Design review of the part shown in the three views and the two pictorial views. Dimensions are in mm from the part's minimum x, y and z. Round coordinates to 2 decimals unless told otherwise and drop trailing zeros. Order: outer loops, then holes, each group sorted by start corner. A loop starts at its lowest first (then second) coordinate and runs counter-clockwise, first axis right, second up.
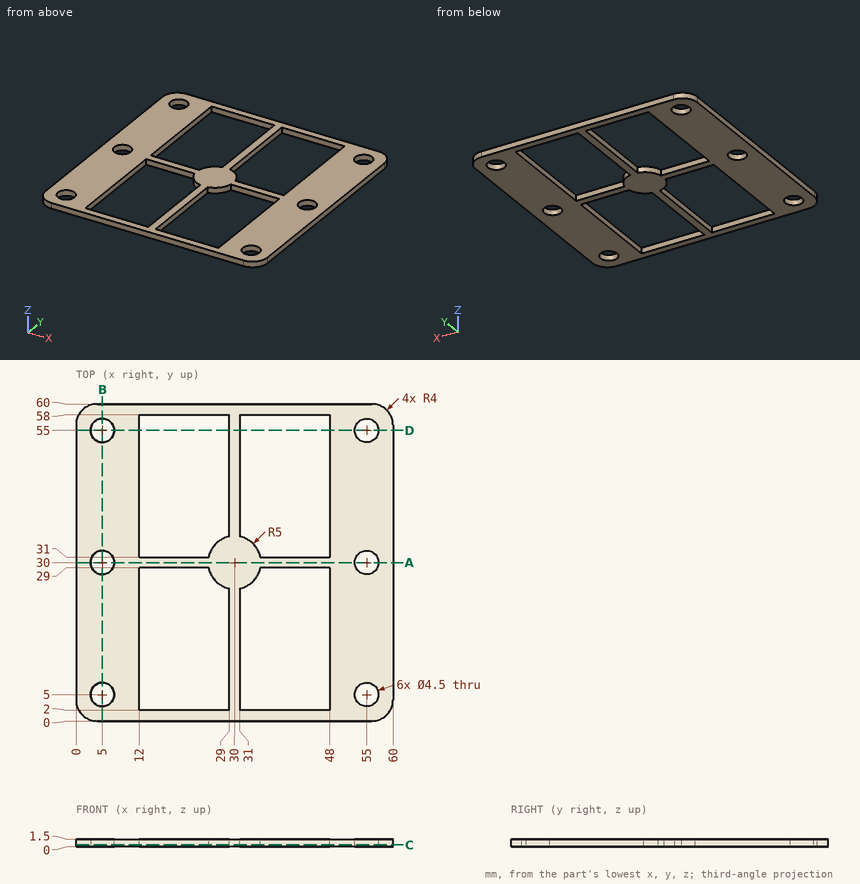
1) Take a section at B-B on x = 5. Give the boundary of the cut face in (y, z).
Results:
outline: (0, 0) - (2.75, 0) - (2.75, 1.5) - (0, 1.5) - close; (7.25, 0) - (27.75, 0) - (27.75, 1.5) - (7.25, 1.5) - close; (32.25, 0) - (52.75, 0) - (52.75, 1.5) - (32.25, 1.5) - close; (57.25, 0) - (60, 0) - (60, 1.5) - (57.25, 1.5) - close
2) Take a section at C-C on z = 0.4. State how many separate pieces and enclosed holes the cut face has, plus the area to 3 significant figures.
Results:
separate pieces: 1
enclosed holes: 10
area: 1,700 mm2
3) Take a section at D-D on y = 55. Give the boundary of the cut face in (x, z).
Results:
outline: (0, 0) - (2.75, 0) - (2.75, 1.5) - (0, 1.5) - close; (7.25, 0) - (12, 0) - (12, 1.5) - (7.25, 1.5) - close; (29, 0) - (31, 0) - (31, 1.5) - (29, 1.5) - close; (48, 0) - (52.75, 0) - (52.75, 1.5) - (48, 1.5) - close; (57.25, 0) - (60, 0) - (60, 1.5) - (57.25, 1.5) - close
4) Take a section at A-A on y = 30. Give the boundary of the cut face in (x, z), plus the area to 3 significant figures.
Results:
outline: (0, 0) - (2.75, 0) - (2.75, 1.5) - (0, 1.5) - close; (7.25, 0) - (52.75, 0) - (52.75, 1.5) - (7.25, 1.5) - close; (57.25, 0) - (60, 0) - (60, 1.5) - (57.25, 1.5) - close
area: 76.5 mm2
5) To check wall thickness, follow line 1 along Y through (x, z) = (5, 0.95); line 2 along Y through (x, z) = (22, 0.45); line 3 along X through (y, z) = (7.5, 1.2). State the ranges of each line that lie inside material, in increasing order.
Results:
line 1: y = 0 to 2.75, 7.25 to 27.75, 32.25 to 52.75, 57.25 to 60
line 2: y = 0 to 2, 29 to 31, 58 to 60
line 3: x = 0 to 12, 29 to 31, 48 to 60
